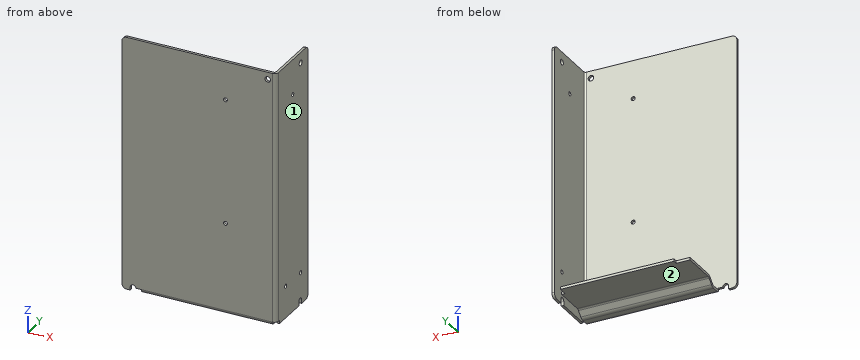
from build123d import *

# Parameters (mm, degrees)
EXTRUDE_THIN1_DEPTH        = 79.5
FILLET1_R                  = 3
EXTRUDE1_DEPTH             = 101.58081328
SKETCH4_W                  = 88.25
SKETCH4_H                  = 2
EXTRUDE2_DEPTH             = 3.5
EXTRUDE_THIN2_START        = -82
EXTRUDE_THIN2_DEPTH        = 82
FILLET2_R                  = 2
SKETCH6_W                  = 2.155687989
SKETCH6_H                  = 5.613141175
SKETCH6_W_2                = 8.683222246
SKETCH6_H_2                = 2.647575272
EXTRUDE3_DEPTH             = 167.425388688
F_3_5_3_5_DIAMETER_HOLE1_D = 3.5
SKETCH9_R                  = 1.75
EXTRUDE4_DEPTH             = 132.046747384
M3_TAPPED_HOLE1_D          = 2.5
M3_TAPPED_HOLE2_D          = 2.5


# Read off the part's stored shape, not the designer's step: Extrude-Thin2
with BuildPart() as part:
    # Sketch1 → Extrude-Thin1 (new, symmetric)
    with BuildSketch(Plane.XY):
        with BuildLine():
            Line((-48.5, 0), (45.9, 0))
            ThreePointArc((45.9, 0), (47.738477631, 0.761522369), (48.5, 2.6))
            Line((48.5, 2.6), (48.5, 38))
            Line((48.5, 38), (46.9, 38))
            Line((46.9, 38), (46.9, 2.6))
            ThreePointArc((46.9, 2.6), (46.607106781, 1.892893219), (45.9, 1.6))
            Line((45.9, 1.6), (-48.5, 1.6))
            Line((-48.5, 1.6), (-48.5, 0))
        make_face()
    extrude(amount=EXTRUDE_THIN1_DEPTH, both=True)

    # Fillet1
    fillet1_edges = [part.edges().sort_by_distance(p)[0] for p in [
        (-48.5, 0.8, 79.5),
        (47.7, 38, 79.5),
        (-48.5, 0.8, -79.5),
        (47.7, 38, -79.5),
    ]]
    fillet(fillet1_edges, radius=FILLET1_R)

    # Sketch3 → Extrude1 (cut, through all)
    with BuildSketch(Plane.XZ):
        with BuildLine():
            Line((-43.25, -81.5), (-43.25, -77.5))
            ThreePointArc((-43.25, -77.5), (-41.5, -75.75), (-39.75, -77.5))
            Line((-39.75, -77.5), (-39.75, -81.5))
            ThreePointArc((-39.75, -81.5), (-41.5, -83.25), (-43.25, -81.5))
        make_face()
    extrude(amount=-EXTRUDE1_DEPTH, mode=Mode.SUBTRACT)

    # Sketch4 → Extrude2 (cut)
    with BuildSketch(Plane.XZ):
        with Locations((4.375, -78.5)):
            Rectangle(SKETCH4_W, SKETCH4_H)
    extrude(amount=-EXTRUDE2_DEPTH, mode=Mode.SUBTRACT)

    # Extrude-Thin2 outline → Extrude-Thin2 (add)
    with BuildSketch(Plane(origin=(45.75, 0, 0), x_dir=(0, 0, -1), z_dir=(1, 0, 0)).offset(EXTRUDE_THIN2_START)):
        with BuildLine():
            Line((77.5, 0), (79.5, 0))
            Line((79.5, 0), (79.5, 6.008831175))
            ThreePointArc((79.5, 6.008831175), (79.225966317, 7.386491532), (78.445584412, 8.554415588))
            Line((78.445584412, 8.554415588), (75.685786438, 11.314213562))
            ThreePointArc((75.685786438, 11.314213562), (75.252240935, 11.96306026), (75.1, 12.728427125))
            Line((75.1, 12.728427125), (75.1, 37))
            Line((75.1, 37), (73.5, 37))
            Line((73.5, 37), (73.5, 12.728427125))
            ThreePointArc((73.5, 12.728427125), (73.774033683, 11.350766768), (74.554415588, 10.182842712))
            Line((74.554415588, 10.182842712), (77.314213562, 7.423044738))
            ThreePointArc((77.314213562, 7.423044738), (77.747759065, 6.77419804), (77.9, 6.008831175))
            Line((77.9, 6.008831175), (77.9, 1.6))
            Line((77.9, 1.6), (77.5, 1.6))
            Line((77.5, 1.6), (77.5, 0))
        make_face()
    extrude(amount=EXTRUDE_THIN2_DEPTH)

    # Fillet2
    fillet2_edges = [part.edges().sort_by_distance(p)[0] for p in [
        (4.75, 0, -79.5),
    ]]
    fillet(fillet2_edges, radius=FILLET2_R)

    # Sketch6 → Extrude3 (cut, through all)
    with BuildSketch(Plane(origin=(0, 0, -75.1), x_dir=(-1, 0, 0), z_dir=(0, 0, -1))):
        with Locations((-44.672156005, 34.193429413)):
            Rectangle(SKETCH6_W, SKETCH6_H)
        with Locations((31.908388877, 35.676212364)):
            Rectangle(SKETCH6_W_2, SKETCH6_H_2)
    extrude(amount=-EXTRUDE3_DEPTH, mode=Mode.SUBTRACT)

    # Ø3.5 (3.5) Diameter Hole1 (through all)
    with Locations(Plane(origin=(0, 1.6, 0), x_dir=(-1, 0, 0), z_dir=(0, 1, 0))):
        with Locations((-43, 75)):
            Hole(F_3_5_3_5_DIAMETER_HOLE1_D / 2)

    # Sketch9 → Extrude4 (cut, through all)
    with BuildSketch(Plane(origin=(48.5, 0, 0), x_dir=(0, 0, -1), z_dir=(1, 0, 0))):
        with Locations((-73, 29)):
            Circle(SKETCH9_R)
        with BuildLine():
            Line((82, 26.75), (77, 26.75))
            ThreePointArc((77, 26.75), (75.25, 28.5), (77, 30.25))
            Line((77, 30.25), (82, 30.25))
            ThreePointArc((82, 30.25), (83.75, 28.5), (82, 26.75))
        make_face()
    extrude(amount=-EXTRUDE4_DEPTH, mode=Mode.SUBTRACT)

    # M3 Tapped Hole1 (through all)
    with Locations(Plane(origin=(48.5, 0, 0), x_dir=(0, 0, -1), z_dir=(1, 0, 0))):
        with Locations((-57.5, 19.5), (59.5, 29), (59.5, 11)):
            Hole(M3_TAPPED_HOLE1_D / 2)

    # M3 Tapped Hole2 (through all)
    with Locations(Plane.XZ):
        with Locations((16.5, 55.5), (16.5, -22.5)):
            Hole(M3_TAPPED_HOLE2_D / 2)


solid = part.part
Geometry check sheet. Reference: the model listing, model coordinates, mm. Face numbers are marked on the shaded views. A direction names the side the tool comes from. Coordinates: 2 decimals unless noted, no trailing zeros. Order: outer loops, then holes, each group sorted by start corner. A loop starts at its lowest first (then second) coordinate and runs counter-clockwise, first axis right, second up. Notation, with made-up numbers: (84.25, 44.25) - (139.25, 44.25) arc R3 cw to (139.25, 48.25) - close; hole circle Ø1 at (44.25, 25). An arc over 180 degrees is marked (long way). Answer in a Markdown table with one row per item. Add a question column.
1) Set-up check for the marked faces 1 and 2: record each of +Z, -Z, +X, -X, +Y, -Y from which the full face is reachable in a straight line by a thin tool's end or side.
2) Cross-section at B-B, the plane y = 16. Record the cut outline in (x, z), then the cut area to 3 significant figures.
3) Cross-section at C-C, the plane x = -14.5. Record the cut outline in (y, z).
4) Material ranges on line 1 along Y through (x, z) = (47.8, -59.5); line 2 along X through (y, z) = (22, 25); line 3 along Y through (x, z) = (-43.5, 30.5), recorded low to high. Write a range as [from, to].
5) Cross-section at A-A, the plane z = -16.5. Record the cut outline in (x, y), then the cut area to 3 significant figures.
6) Gauge pin test, flat ends, axial feed: P1, Ø1, axis at x = -10.5, z = 42.5, coming from the +Y side; P2, Ø1.3, axis at x = -2, z = -74.5, coming from the +Y side; P3, Ø1.8, axis at x = 48, z = -78, coming from the -Y side. Record the tip position at first contact, or that the pin passes through.
Check result:
| question | item | result |
|---|---|---|
| 1 | face 1 | +Z, -Z, +X, +Y, -Y |
| 1 | face 2 | -Z, -X, +Y |
| 2 | outline | (-36.25, -75.1) - (45.75, -75.1) - (45.75, -73.5) - (-36.25, -73.5) - close; (46.9, -79.5) - (48.5, -79.5) - (48.5, 79.5) - (46.9, 79.5) - close |
| 2 | area | 386 mm² |
| 3 | outline | (0, -77.5) arc R2 ccw to (2, -79.5) - (6.01, -79.5) arc R3.6 ccw to (8.55, -78.45) - (11.31, -75.69) arc R2 cw to (12.73, -75.1) - (37, -75.1) - (37, -73.5) - (12.73, -73.5) arc R3.6 ccw to (10.18, -74.55) - (7.42, -77.31) arc R2 cw to (6.01, -77.9) - (1.6, -77.9) - (1.6, 79.5) - (0, 79.5) - close |
| 4 | line 1 | y = [0.83, 9.75], [12.25, 27.75], [30.25, 38] |
| 4 | line 2 | x = [46.9, 48.5] |
| 4 | line 3 | y = [0, 1.6] |
| 5 | outline | (-48.5, 0) - (45.9, 0) arc R2.6 ccw to (48.5, 2.6) - (48.5, 38) - (46.9, 38) - (46.9, 2.6) arc R1 cw to (45.9, 1.6) - (-48.5, 1.6) - close |
| 5 | area | 212 mm² |
| 6 | P1 | stops at y = 1.6 |
| 6 | P2 | stops at y = 37 |
| 6 | P3 | stops at y = 0.38 |
